Design review of the part shown in the three views and the two pictorial views. Dimensions are in mm from the part's minimum x, y and z. A direction names the side the tool comes from. Coordinates: 2 decimals unless noted, no trailing zeros. Loops run counter-clockwise (first coordinate to the right, second up) from the corner with the lowest first, then second, coordinate; pieces in that order, holes last. Notation, with made-up numbers: (61.5, 23) -> (115.5, 23) arc R16 cw to (115.5, 54) -> close; hole circle Ø9 at (32.5, 85). An arc over 180 degrees is marked (long way). One line per item, written item: value.
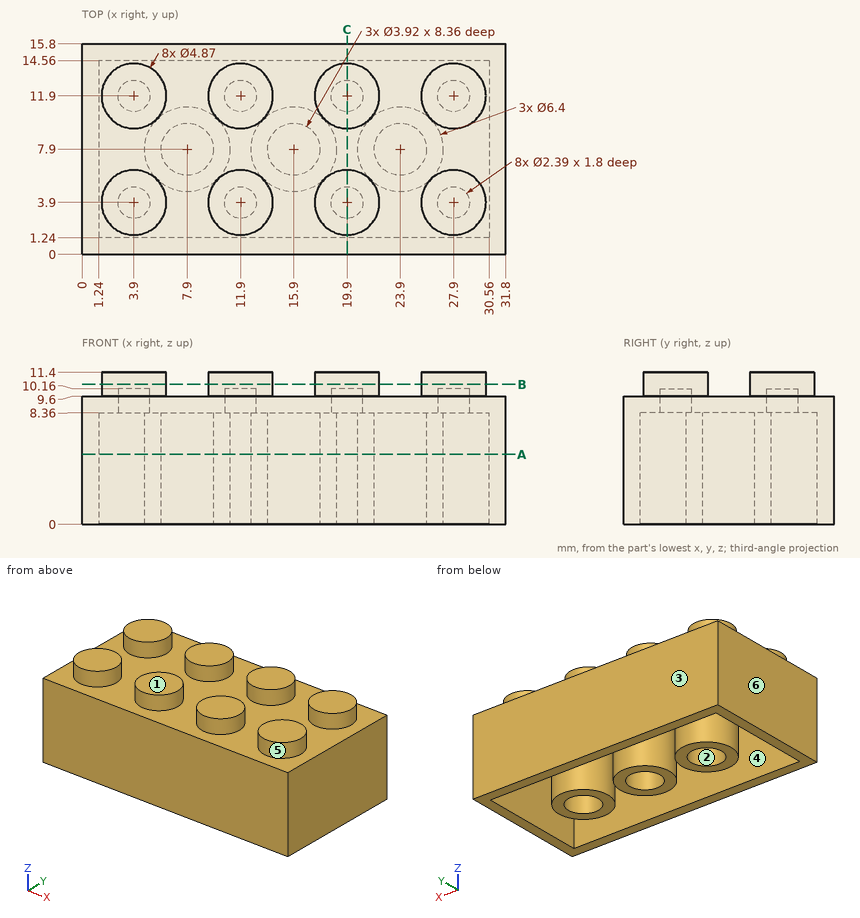
1. Take a section at C-C, the plane x = 19.9. Give the boundary of the cut face in (y, z) (3 decimals), and give its area (3 significant figures).
Return value:
outline: (0, 0) -> (1.24, 0) -> (1.24, 8.36) -> (2.705, 8.36) -> (2.705, 10.16) -> (5.095, 10.16) -> (5.095, 8.36) -> (10.705, 8.36) -> (10.705, 10.16) -> (13.095, 10.16) -> (13.095, 8.36) -> (14.56, 8.36) -> (14.56, 0) -> (15.8, 0) -> (15.8, 9.6) -> (14.335, 9.6) -> (14.335, 11.4) -> (9.465, 11.4) -> (9.465, 9.6) -> (6.335, 9.6) -> (6.335, 11.4) -> (1.465, 11.4) -> (1.465, 9.6) -> (0, 9.6) -> close
area: 49.3 mm2
2. For the marked faces 4, 5 and 6, list the 3-axis set-ups (+Z, -Z, +X, -X, +Y, -Y) from which the entire face can be reached by the end or side of a thin tool; tool diameter is ignored.
Return value:
face 4: -Z
face 5: +Z
face 6: +Z, -Z, -X, +Y, -Y
3. Take a section at B-B, the plane z = 10.5. Give the boundary of the cut face in (x, y) (3 decimals), and give its area (3 significant figures).
Return value:
outline: circle Ø4.87 at (3.9, 3.9); circle Ø4.87 at (3.9, 11.9); circle Ø4.87 at (11.9, 3.9); circle Ø4.87 at (11.9, 11.9); circle Ø4.87 at (19.9, 3.9); circle Ø4.87 at (19.9, 11.9); circle Ø4.87 at (27.9, 3.9); circle Ø4.87 at (27.9, 11.9)
area: 149 mm2
4. The part is to be moulded in two halves that separate along Y. For the marked faces 1, 2 and 3, say which applies: pulls with the +Y half, pulls with the -Y half, needs draft (parallel to the pull), parting line crosses it, or undercut.
Return value:
face 1: needs draft
face 2: undercut
face 3: pulls with the +Y half
5. Take a section at A-A, the plane z = 5.25. Give the boundary of the cut face in (x, y), and give its area (3 significant figures).
Return value:
outline: (0, 0) -> (31.8, 0) -> (31.8, 15.8) -> (0, 15.8) -> close; circle Ø6.4 at (7.9, 7.9); circle Ø6.4 at (15.9, 7.9); circle Ø6.4 at (23.9, 7.9); hole (1.24, 1.24) -> (30.56, 1.24) -> (30.56, 14.56) -> (1.24, 14.56) -> close; hole circle Ø3.92 at (7.9, 7.9); hole circle Ø3.92 at (15.9, 7.9); hole circle Ø3.92 at (23.9, 7.9)
area: 172 mm2
6. To check wall thickness, follow probe 1 along X at (y, z) = (4, 10.25); probe 2 along Y at (x, z) = (7.9, 2.75); probe 3 along X at (y, z) = (3.9, 8.8) (3 decimals). State the ranges of each line that lie inside material, in increasing order. Write a range as from..to.
Return value:
probe 1: x = 1.47..6.33, 9.47..14.33, 17.47..22.33, 25.47..30.33
probe 2: y = 0..1.24, 4.7..5.94, 9.86..11.1, 14.56..15.8
probe 3: x = 0..2.705, 5.095..10.705, 13.095..18.705, 21.095..26.705, 29.095..31.8
7. Insertion check: pin 1 Ø2.5 at (x, y) = (19.9, 11.9) entering from -Z; pin 2 Ø2 at (x, y) = (15.5, 9) entering from +Z; pin 3 Ø1.9 at (x, y) = (19.9, 3.9) entering from -Z. Each pin has a flat end and moves straight along its axis. Give the tip position at first contact, or say it passes through.
Return value:
pin 1: stops at z = 8.36
pin 2: stops at z = 9.6
pin 3: stops at z = 10.16
